```python
from build123d import *

# Parameters (mm, degrees)
SKETCH1_R                = 50
SKETCH1_R_2              = 5
BOSS_EXTRUDE1_DEPTH      = 5
SKETCH2_R                = 1.2
SKETCH2_R_2              = 1.225
SKETCH2_R_3              = 5.05
SKETCH2_R_4              = 1.015
CUT_EXTRUDE1_DEPTH       = 10
SKETCH5_R                = 5
SKETCH5_R_2              = 1.015
BOSS_EXTRUDE2_DEPTH      = 6
SKETCH9_R                = 2.357259082
BOSS_EXTRUDE4_DEPTH      = 1
FILLET1_R                = 1
SKETCH10_R               = 1.5
CUT_EXTRUDE3_DEPTH       = 2.2
CUT_EXTRUDE3_DEPTH_BACK  = 16
CUT_EXTRUDE6_DEPTH       = 0.5
CUT_EXTRUDE7_DEPTH       = 10
CUT_EXTRUDE9_DEPTH       = 10
CUT_EXTRUDE9_DEPTH_BACK  = 10
SKETCH17_R               = 5.5
CUT_EXTRUDE10_DEPTH      = 10
CUT_EXTRUDE10_DEPTH_BACK = 10
SKETCH18_R               = 2.25
CUT_EXTRUDE11_DEPTH      = 2.2


with BuildPart() as part:
    # Sketch1 → Boss-Extrude1 (new body)
    with BuildSketch(Plane(origin=(0, 0, 0), x_dir=(1, 0, 0), z_dir=(0, 1, 0))):
        Circle(SKETCH1_R)
        with Locations((-7.573934673, -17.06033615)):
            Circle(SKETCH1_R_2, mode=Mode.SUBTRACT)
    extrude(amount=BOSS_EXTRUDE1_DEPTH)

    # Sketch2 → Cut-Extrude1 (cut)
    with BuildSketch(Plane(origin=(0, 5, 0), x_dir=(1, 0, 0), z_dir=(0, 1, 0))):
        with Locations((26.030814012, 7.899159566)):
            Circle(SKETCH2_R)
        with Locations((17.087578103, 21.16635714)):
            Circle(SKETCH2_R)
        with Locations((13.062426036, 8.805202225)):
            Circle(SKETCH2_R_2)
        with Locations((21.559196058, 14.532758353)):
            Circle(SKETCH2_R_3)
        with Locations((8.320757608, 18.248434254)):
            Circle(SKETCH2_R_4)
    extrude(amount=-CUT_EXTRUDE1_DEPTH, mode=Mode.SUBTRACT)

    # Sketch5 → Boss-Extrude2 (add)
    with BuildSketch(Plane(origin=(0, 5, 0), x_dir=(1, 0, 0), z_dir=(0, 1, 0))):
        with Locations((-7.55311225, 14.331451264)):
            Circle(SKETCH5_R)
        with Locations((-7.55311225, 14.331451264)):
            Circle(SKETCH5_R_2, mode=Mode.SUBTRACT)
    extrude(amount=BOSS_EXTRUDE2_DEPTH)

    # Sketch9 → Boss-Extrude4 (add)
    with BuildSketch(Plane.XZ):
        with Locations((8.320757608, -18.248434254)):
            Circle(SKETCH9_R)
    extrude(amount=-BOSS_EXTRUDE4_DEPTH)

    # Fillet1
    fillet1_edges = [part.edges().sort_by_distance(p)[0] for p in [
        (-50, 5, 0),
    ]]
    fillet(fillet1_edges, radius=FILLET1_R)

    # Sketch10 → Cut-Extrude3 (cut, two sides)
    with BuildSketch(Plane(origin=(0, 5, 0), x_dir=(1, 0, 0), z_dir=(0, 1, 0))) as cut_extrude3_sk:
        with Locations((0, 37.8)):
            Circle(SKETCH10_R)
        with Locations((-32.735760263, -18.9)):
            Circle(SKETCH10_R)
        with Locations((32.735760263, -18.9)):
            Circle(SKETCH10_R)
    extrude(amount=CUT_EXTRUDE3_DEPTH, mode=Mode.SUBTRACT)
    extrude(cut_extrude3_sk.sketch, amount=-CUT_EXTRUDE3_DEPTH_BACK, mode=Mode.SUBTRACT)

    # Sketch12 → Cut-Extrude6 (cut)
    with BuildSketch(Plane.XZ):
        with BuildLine():
            Line((-21.313834783, 24.76213107), (-34.538834783, 1.855759139))
            ThreePointArc((-34.538834783, 1.855759139), (-35.038336896, -1.938336086), (-32.708707764, -4.974367879))
            Line((-32.708707764, -4.974367879), (-14.089161583, -15.724367879))
            ThreePointArc((-14.089161583, -15.724367879), (-10.295066357, -16.223869992), (-7.259034564, -13.894240861))
            Line((-7.259034564, -13.894240861), (5.965965436, 9.01213107))
            ThreePointArc((5.965965436, 9.01213107), (0.201065327, 30.527031179), (-21.313834783, 24.76213107))
        make_face()
    extrude(amount=-CUT_EXTRUDE6_DEPTH, mode=Mode.SUBTRACT)

    # Sketch13 → Cut-Extrude7 (cut)
    with BuildSketch(Plane(origin=(0, 5, 0), x_dir=(1, 0, 0), z_dir=(0, 1, 0))):
        with BuildLine():
            Line((32.816836472, -6.07169605), (21.984996749, -21.138640776))
            ThreePointArc((21.984996749, -21.138640776), (16.391033491, -22.978825985), (12.925236211, -18.21784334))
            Line((12.925236211, -18.21784334), (12.931687147, -3.407234286))
            ThreePointArc((12.931687147, -3.407234286), (14.35531099, 0.084802692), (17.813324255, 1.589186743))
            Line((17.813324255, 1.589186743), (28.638713042, 1.845522414))
            ThreePointArc((28.638713042, 1.845522414), (33.179093412, -0.819461796), (32.816836472, -6.07169605))
        make_face()
    extrude(amount=-CUT_EXTRUDE7_DEPTH, mode=Mode.SUBTRACT)

    # Sketch16 → Cut-Extrude9 (cut, two sides)
    with BuildSketch(Plane.XZ.offset(-0.5)) as cut_extrude9_sk:
        with BuildLine():
            Line((-12.984156175, 14.705600426), (-13.719701132, 11.95882482))
            ThreePointArc((-13.719701132, 11.95882482), (-13.693758532, 7.802544191), (-11.54963643, 4.241914739))
            Line((-11.54963643, 4.241914739), (-10.842839117, 3.568938111))
            ThreePointArc((-10.842839117, 3.568938111), (-9.907482144, -2.457917187), (-15.493944375, -4.905225341))
            Line((-15.493944375, -4.905225341), (-19.004093622, -4.034917019))
            ThreePointArc((-19.004093622, -4.034917019), (-20.457115896, -3.417911536), (-21.645362284, -2.3786618))
            Line((-21.645362284, -2.3786618), (-25.653320737, 2.441392154))
            ThreePointArc((-25.653320737, 2.441392154), (-26.807383132, 5.519886283), (-25.80025353, 8.649531003))
            Line((-25.80025353, 8.649531003), (-19.012059198, 17.647148968))
            ThreePointArc((-19.012059198, 17.647148968), (-14.786139745, 18.659973084), (-12.984156175, 14.705600426))
        make_face()
    extrude(amount=CUT_EXTRUDE9_DEPTH, mode=Mode.SUBTRACT)
    extrude(cut_extrude9_sk.sketch, amount=-CUT_EXTRUDE9_DEPTH_BACK, mode=Mode.SUBTRACT)

    # Sketch17 → Cut-Extrude10 (cut, two sides)
    with BuildSketch(Plane.XZ.offset(-0.5)) as cut_extrude10_sk:
        Circle(SKETCH17_R)
    extrude(amount=CUT_EXTRUDE10_DEPTH, mode=Mode.SUBTRACT)
    extrude(cut_extrude10_sk.sketch, amount=-CUT_EXTRUDE10_DEPTH_BACK, mode=Mode.SUBTRACT)

    # Sketch18 → Cut-Extrude11 (cut)
    with BuildSketch(Plane(origin=(0, 5, 0), x_dir=(1, 0, 0), z_dir=(0, 1, 0))):
        with Locations((17.087578103, 21.16635714)):
            Circle(SKETCH18_R)
        with Locations((26.030814012, 7.899159566)):
            Circle(SKETCH18_R)
    extrude(amount=-CUT_EXTRUDE11_DEPTH, mode=Mode.SUBTRACT)


solid = part.part
```
The listing builds one solid part. Answer for the finished solid, in the listing's coordinates (mm). A direction names the side the tool comes from. Round coordinates to 2 decimals unless told otherwise and drop trailing zeros. Write each loop counter-clockwise with the first axis right and the second up, starting at its lowest first coordinate (ties: lowest second). Pieces come first, ordered by that corner, then holes. Notation, with made-up numbers: (84.25, 64.5) -> (105.25, 64.5) arc R15 ccw to (105.25, 80.5) -> close; hole circle Ø2 at (6, -21.5). An arc over 180 degrees is marked (long way). Write item = value, one per line.
1) Section A-A on z = 0 is taken. Write down the section's boundary in (x, y).
Check values:
outline = (-50, 0) -> (-35.17, 0) -> (-35.17, 0.5) -> (-23.62, 0.5) -> (-23.62, 5) -> (-49, 5) arc R1 ccw to (-50, 4) -> close; (-9.29, 0.5) -> (-5.5, 0.5) -> (-5.5, 5) -> (-9.29, 5) -> close; (5.5, 0) -> (14.27, 0) -> (14.27, 5) -> (5.5, 5) -> close; (32.64, 0) -> (50, 0) -> (50, 4) arc R1 ccw to (49, 5) -> (32.64, 5) -> close
2) Which of the six approach directions +Z, -Z, +X, -X, +Y, -Y give full straight-line access (tool end or side, diameter ignored) to faces 4 (the flat face through (4.615, 0.246, 6.673)), 5 (the flat face through (18, 2.8, -20)), 6 (the cylindrical face through (16.475, 2.535, 23.005))?
Check values:
face_4 = -Y
face_5 = +Y
face_6 = +Y, -Y
3) Straight lines are drawn through the part: line 1 along Z through (x, y) = (0, 1.7); line 2 along X through (y, z) = (2.25, 9); line 3 along Y through (x, z) = (30.5, 10.5). For each, find the intervals that lie inside material, in ascending order. Write a range as [from, to].
Check values:
line_1 = [-50, -39.3], [-36.3, -5.5], [5.5, 50]
line_2 = [-49.18, -25.54], [-13.93, 12.93], [30.71, 49.18]
line_3 = [0, 5]
4) For a pull along Z with two mould halves and no side action, classify faces 1 (the flat face through (-8, 11, -13)), 2 (the cylindrical face through (-14.85, 2.72, 18.69)), 3 (the cylindrical face through (-8.2, 7.96, -19.29)) as released by +Z, released by -Z, zero draft, split by the parting line, or undercut.
Check values:
face_1 = zero draft
face_2 = undercut
face_3 = split by the parting line
5) Section B-B on x = 0 is taken. Write down the section's boundary in (y, z), plus the area to 3 significant figures.
Check values:
outline = (0, -50) -> (4, -50) arc R1 ccw to (5, -49) -> (5, -39.3) -> (0, -39.3) -> close; (0, -36.3) -> (5, -36.3) -> (5, -5.5) -> (0, -5.5) -> close; (0, 30.64) -> (0.5, 30.64) -> (0.5, 5.5) -> (5, 5.5) -> (5, 49) arc R1 ccw to (4, 50) -> (0, 50) -> close
area = 417 mm²
6) Given pin 1 (16 mm diameter, centred on x = -7.57, z = 17.06, fed in from +Y); pin 2 (2.5 mm diameter, centred on y = 2.5, z = 8, fed in from +X); pin 3 (6 mm diameter, centred on x = 31, y = 7.5, fed in from -Z), each flat-ended and moving along its own axis, determine where each tip first touches the part or whether it passes through.
Check values:
pin_1 = 5
pin_2 = 49.54
pin_3 = -39.73
7) Section C-C on y = 6.25 is taken. Write down the section's boundary in (x, z) (3 decimals).
Check values:
outline = circle Ø10 at (-7.553, -14.331); hole circle Ø2.03 at (-7.553, -14.331)
